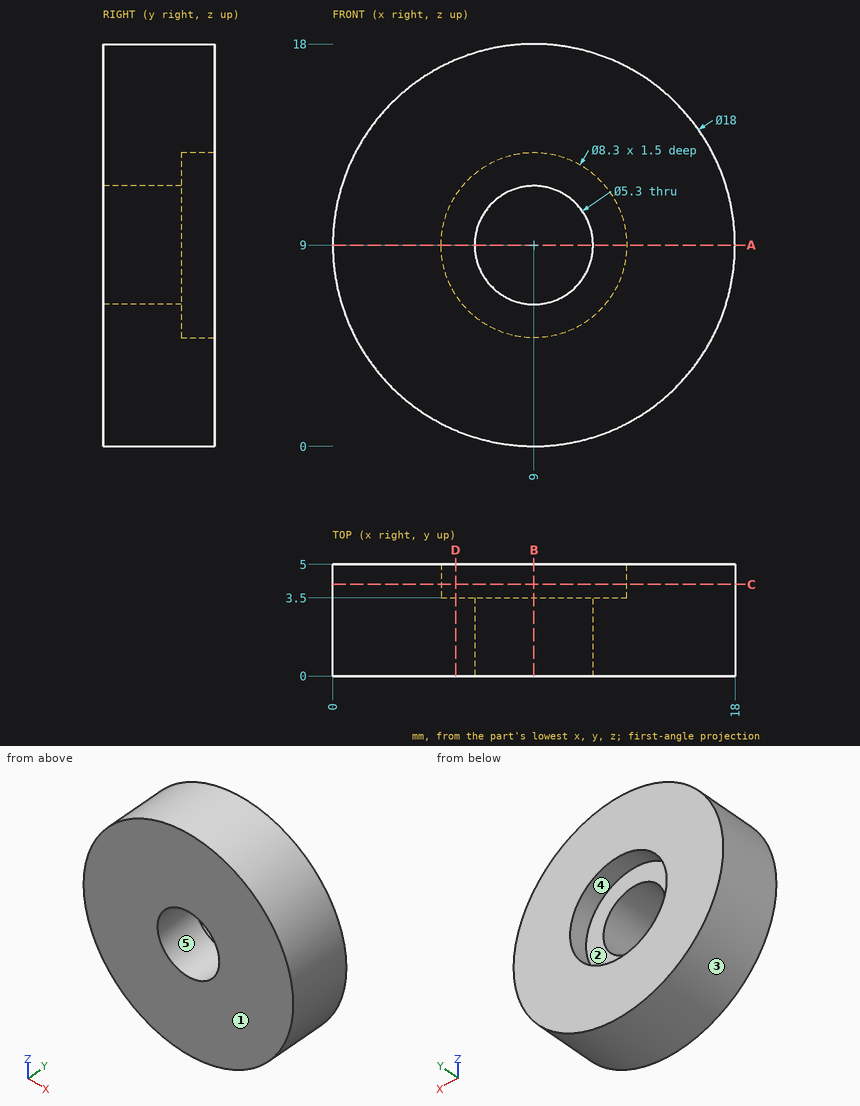
The figure shows three views and two pictorial views of one solid part (mm, origin at its lowest corner). Answer the questions. A direction names the side the tool comes from. Give positions to 0.01 mm unless a question says otherwise; leave off trailing zeros. Order: outer loops, then holes, each group sorted by start corner. A loop starts at its lowest first (then second) coordinate and runs counter-clockwise, first axis right, second up. Notation, with made-up numbers: (65, 48) -> (95, 48) arc R6 ccw to (95, 58) -> close; hole circle Ø4 at (55.25, 1). An arc over 180 degrees is marked (long way). Answer as CSV lines item,"result". Start each with the question number.
(1) Which of the six approach directions +Z, -Z, +X, -X, +Y, -Y give full straight-line access (tool end or side, diameter ignored) to the marked faces 4 and 5?
(2) Section B-B, the plane x = 9 is taken. Write down the section's boundary in (y, z).
(3) Section D-D, the plane x = 5.5 is taken. Write down the section's boundary in (y, z).
(4) Section C-C, the plane y = 4.1 is taken. Write down the section's boundary in (x, z).
(5) For a pull along X with two mould halves and no side action, classify the marked faces 1, 2 and 3 as released by +X, released by -X, zero draft, split by the parting line, or undercut.
(6) Section A-A, the plane z = 9 is taken. Write down the section's boundary in (x, y), plus the area to 3 significant figures.
(7) Each of these flat-tipped pins is pushed along its axis until it touches: pin 1 Ø1 at (y, z) = (1.5, 4.5) entering from +X; pin 2 Ø3 at (x, z) = (9, 9) entering from -Y; pin 3 Ø1 at (y, z) = (4.5, 11.5) entering from +X; pin 4 Ø4 at (x, z) = (9, 7.5) entering from +Y. Where does it stop, or does it pass through?
(8) Consider line 1 along Z through (x, y) = (9, 2.4); line 2 along Y through (x, z) = (5.75, 6.5); line 3 along Z through (x, y) = (11.5, 4). Determine where each line is inside the solid, lowest interval first.
Entries:
1,face 4,"+Y"
1,face 5,"+Y, -Y"
2,outline,"(0, 0) -> (5, 0) -> (5, 4.85) -> (3.5, 4.85) -> (3.5, 6.35) -> (0, 6.35) -> close; (0, 11.65) -> (3.5, 11.65) -> (3.5, 13.15) -> (5, 13.15) -> (5, 18) -> (0, 18) -> close"
3,outline,"(0, 0.71) -> (5, 0.71) -> (5, 6.77) -> (3.5, 6.77) -> (3.5, 11.23) -> (5, 11.23) -> (5, 17.29) -> (0, 17.29) -> close"
4,outline,"circle Ø18 at (9, 9); hole circle Ø8.3 at (9, 9)"
5,face 1,"zero draft"
5,face 2,"undercut"
5,face 3,"split by the parting line"
6,outline,"(0, 0) -> (6.35, 0) -> (6.35, 3.5) -> (4.85, 3.5) -> (4.85, 5) -> (0, 5) -> close; (11.65, 0) -> (18, 0) -> (18, 5) -> (13.15, 5) -> (13.15, 3.5) -> (11.65, 3.5) -> close"
6,area,"59.0 mm²"
7,pin 1,"x = 17.06"
7,pin 2,"through"
7,pin 3,"x = 17.77"
7,pin 4,"y = 3.5"
8,line 1,"0 to 6.35, 11.65 to 18"
8,line 2,"0 to 3.5"
8,line 3,"0.35 to 5.69, 12.31 to 17.65"
